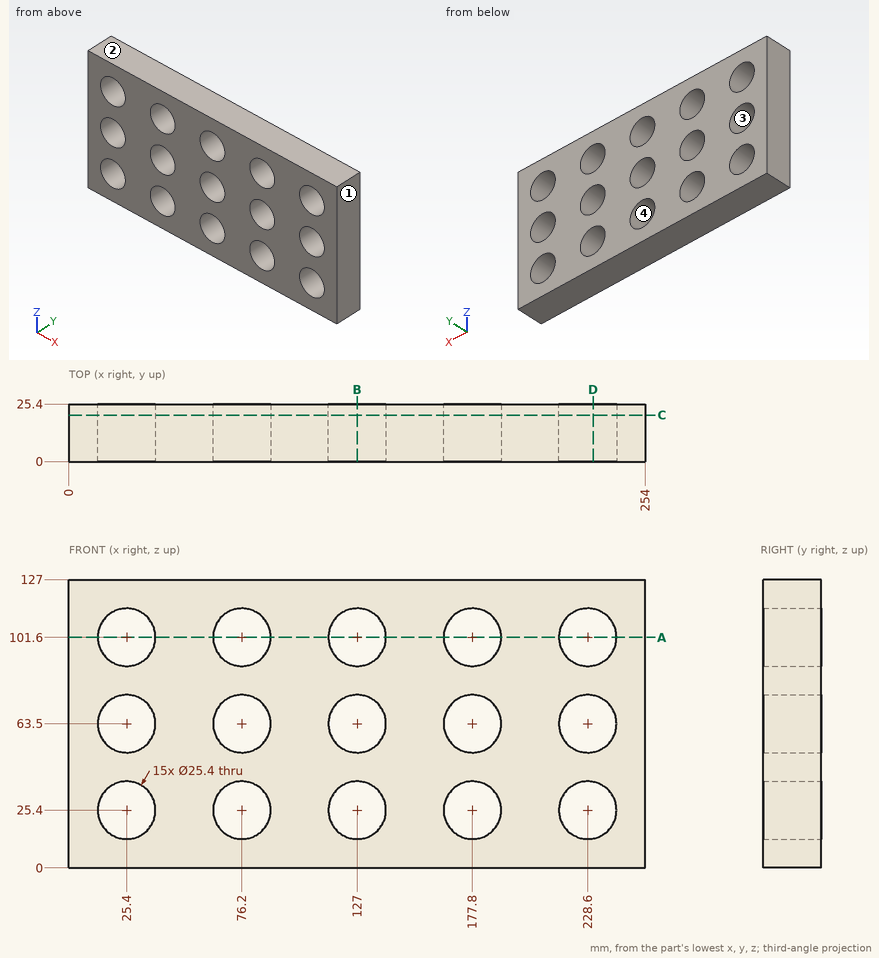
Geometry: see drawing. Coordinates: mm, zero at the bounding-box minimum. Round coordinates to 2 decimals unless told otherwise and drop trailing zeros. Write each loop counter-clockwise with the first axis right and the second up, starting at its lowest first coordinate (ties: lowest second). Pieces come first, ordered by that corner, then holes.
Item 1: Mould query, pull axis X, two halves, no side actions, for the marked faces 1, 2, 3 and 4. Classes: +X half, -X half, draft (parallel to the pull), parting line (faces both ways), or undercut.
Item 2: Section query B-B (x = 127). Return loops of the section in (y, z).
Item 3: Section query D-D (x = 231). Return loops of the section in (y, z), plus the area to 3 significant figures.
Item 4: Section query C-C (y = 20.5). Give the number of separate pieces and of enclosed holes in the cut face, plus the area to 3 significant figures.
Item 5: Section query A-A (z = 101.6). Return loops of the section in (x, y).
Item 6: Material intervals for L1, parallel to Z at x = 228.6, y = 17.25; L2, parallel to Z at x = 28, y = 18; L3, parallel to X at y = 11.75, z = 24.5, sorted ascending.
Completed:
1. face 1: +X half
1. face 2: draft
1. face 3: undercut
1. face 4: undercut
2. outline: (0, 0) - (25.4, 0) - (25.4, 12.7) - (0, 12.7) - close; (0, 38.1) - (25.4, 38.1) - (25.4, 50.8) - (0, 50.8) - close; (0, 76.2) - (25.4, 76.2) - (25.4, 88.9) - (0, 88.9) - close; (0, 114.3) - (25.4, 114.3) - (25.4, 127) - (0, 127) - close
3. outline: (0, 0) - (25.4, 0) - (25.4, 12.93) - (0, 12.93) - close; (0, 37.87) - (25.4, 37.87) - (25.4, 51.03) - (0, 51.03) - close; (0, 75.97) - (25.4, 75.97) - (25.4, 89.13) - (0, 89.13) - close; (0, 114.07) - (25.4, 114.07) - (25.4, 127) - (0, 127) - close
3. area: 1,330 mm2
4. separate pieces: 1
4. enclosed holes: 15
4. area: 24,700 mm2
5. outline: (0, 0) - (12.7, 0) - (12.7, 25.4) - (0, 25.4) - close; (38.1, 0) - (63.5, 0) - (63.5, 25.4) - (38.1, 25.4) - close; (88.9, 0) - (114.3, 0) - (114.3, 25.4) - (88.9, 25.4) - close; (139.7, 0) - (165.1, 0) - (165.1, 25.4) - (139.7, 25.4) - close; (190.5, 0) - (215.9, 0) - (215.9, 25.4) - (190.5, 25.4) - close; (241.3, 0) - (254, 0) - (254, 25.4) - (241.3, 25.4) - close
6. L1: z = 0 to 12.7, 38.1 to 50.8, 76.2 to 88.9, 114.3 to 127
6. L2: z = 0 to 12.97, 37.83 to 51.07, 75.93 to 89.17, 114.03 to 127
6. L3: x = 0 to 12.73, 38.07 to 63.53, 88.87 to 114.33, 139.67 to 165.13, 190.47 to 215.93, 241.27 to 254
